Design review of the part built by this model. Coordinates are the model's own, in mm. Coordinates: 2 decimals unless noted, no trailing zeros. Write each loop counter-clockwise with the first axis right and the second up, starting at its lowest first coordinate (ties: lowest second). Pieces come first, ordered by that corner, then holes. Notation, with made-up numbers: (25.25, -37) -> (39.25, -37) arc R15 ccw to (39.25, -12) -> close; hole circle Ø3 at (-15, -35.75). An arc over 180 degrees is marked (long way). One line per question, with ' | ' between items. Start each with the question number.
Q1. Draft analysis for pull direction Z (two halves, no side actions). For faces 1 (the flat face through (0, 46, 62.5)), 2 (the flat face through (-6, 15, -6)), 3 (the cylindrical face through (-3.083, 7.605, 7.436)), 4 (the flat face through (-0.18, 33.92, 37.15)), state which applies: pulls with the +Z half, pulls with the -Z half, needs draft (parallel to the pull), parting line crosses it, or undercut.
Q2. Add section B-B on z = 0. State the section outline as (x, y) points.
Q3. Wall thickness on probe 1 along X at (y, z) = (7, 0); probe 2 along Y at (x, z) = (-9.25, -2.5); probe 3 along Y at (x, z) = (5, 41.5): over which ranges is each line inside the solid? List them lowest first.
Q4. For P1, Ø1.5, axis at x = 9.5, z = 1, coming from the +Y side; P2, Ø2, axis at x = 5, y = 27, coming from the -Z side; P3, Ø2, axis at x = -3, y = 5.5, coming from the +Z side; P4, Ø9.5, axis at x = 0, z = 0, coming from the +Y side, all flat-tipped, find the tip position at first contact; note any pin that passes through.
Q5. Add section C-C on x = 10. State the section outline as (y, z) points, and give its area (4 significant figures).
Q6. Add section A-A on x = 0. State the section outline as (y, z) points, and give its area (4 significant figures).
Q7. Add section D-D on x = -3.75. State the section outline as (y, z) points.
from build123d import *

# Parameters (mm, degrees)
SKETCH_1_W          = 25
SKETCH_1_H          = 25
EXTRUDE_1_DEPTH     = 15
SKETCH_2_R          = 8.05
CUT_EXTRUDE_1_DEPTH = 24.184046239
EXTRUDE_2_DEPTH     = 25


with BuildPart() as part:
    # 草图1 → 凸台-拉伸1 (new body)
    with BuildSketch(Plane(origin=(0, 0, 0), x_dir=(1, 0, 0), z_dir=(0, 1, 0))):
        Rectangle(SKETCH_1_W, SKETCH_1_H)
    extrude(amount=EXTRUDE_1_DEPTH)

    # 草图2 → 切除-拉伸1 (cut, through all)
    with BuildSketch(Plane(origin=(0, 15, 0), x_dir=(1, 0, 0), z_dir=(0, 1, 0))):
        with Locations(Location((0, 0, 0), (0, 0, 270))):
            Circle(SKETCH_2_R)
    extrude(amount=-CUT_EXTRUDE_1_DEPTH, mode=Mode.SUBTRACT)

    # 草图3 → 凸台-拉伸2 (add)
    with BuildSketch(Plane.ZY.offset(12.5)):
        Polygon((12.5, 15), (62.5, 53.379349155), (62.5, 38.379349155), (12.5, 0), align=None)
    extrude(amount=-EXTRUDE_2_DEPTH)


solid = part.part
Output values:
1) face 1: pulls with the +Z half | face 2: needs draft | face 3: undercut | face 4: pulls with the -Z half
2) outline: (-12.5, 0) -> (-8.05, 0) -> (-8.05, 15) -> (-12.5, 15) -> close; (8.05, 0) -> (12.5, 0) -> (12.5, 15) -> (8.05, 15) -> close
3) probe 1: x = -12.5 to -8.05, 8.05 to 12.5 | probe 2: y = 0 to 15 | probe 3: y = 22.26 to 37.26
4) P1: stops at y = 15 | P2: stops at z = 26.83 | P3: stops at z = 20.97 | P4: passes through
5) outline: (0, -12.5) -> (15, -12.5) -> (15, 12.5) -> (53.38, 62.5) -> (38.38, 62.5) -> (0, 12.5) -> close | area: 1,125 mm2
6) outline: (0, -12.5) -> (15, -12.5) -> (15, -8.05) -> (0, -8.05) -> close; (0, 8.05) -> (15, 8.05) -> (15, 12.5) -> (53.38, 62.5) -> (38.38, 62.5) -> (0, 12.5) -> close | area: 883.5 mm2
7) outline: (0, -12.5) -> (15, -12.5) -> (15, -7.12) -> (0, -7.12) -> close; (0, 7.12) -> (15, 7.12) -> (15, 12.5) -> (53.38, 62.5) -> (38.38, 62.5) -> (0, 12.5) -> close
